```python
from build123d import *

# Parameters (mm, degrees)
F3_DEPTH = 30
F4_DEPTH = 30
F5_DEPTH = 30


with BuildPart() as f3:
    # F0 (on Top) → F3 (new body, symmetric)
    with BuildSketch(Plane.XY):
        Polygon((17.320508, 30), (-17.320508, 30), (-34.641016, 0), (-17.320508, -30), (17.320508, -30), (34.641016, 0), align=None)
    extrude(amount=F3_DEPTH, both=True)

    # F1 (on Right) → F4 (intersect, symmetric)
    with BuildSketch(Plane.YZ):
        Polygon((30, -17.320508), (30, 17.320508), (0, 34.641016), (-30, 17.320508), (-30, -17.320508), (0, -34.641016), align=None)
    extrude(amount=F4_DEPTH, both=True, mode=Mode.INTERSECT)

    # F2 (on Front) → F5 (intersect, symmetric)
    with BuildSketch(Plane.XZ):
        Polygon((17.320508, 30), (-17.320508, 30), (-34.641016, 0), (-17.320508, -30), (17.320508, -30), (34.641016, 0), align=None)
    extrude(amount=F5_DEPTH, both=True, mode=Mode.INTERSECT)


solid = f3.part
```
Model file for the job. Use its own axes, mm. Give positions to 0.01 mm unless a question says otherwise; leave off trailing zeros. Order: outer loops, then holes, each group sorted by start corner. A loop starts at its lowest first (then second) coordinate and runs counter-clockwise, first axis right, second up.
1) Saw through at A-A, the plane z = 3. Write the cut outline in (x, y).
2) Pin check, flat tips, straight feed: pin 1 (5 mm diameter, centred on x = 19.5, y = -19, fed in from +Z); pin 2 (4 mm diameter, centred on y = -13.5, z = -3.5, fed in from -X); pin 3 (3 mm diameter, centred on x = 8, y = -11.5, fed in from +Z). Stop position of each tip, or through.
3) Wall check: probe 1 along Y at (x, z) = (-20, 3); probe 2 along Y at (x, z) = (18, -21.5); probe 3 along X at (y, z) = (-5, 20). Give the ranges that are in metal, low to high.
4) Saw through at D-D, the plane z = 26. Write the cut outline in (x, y).
5) Saw through at C-C, the plane x = -23. Write the cut outline in (y, z), then the cut area to 3 significant figures.
Computed:
1. outline: (-30, -8.04) - (-17.32, -30) - (17.32, -30) - (30, -8.04) - (30, 8.04) - (17.32, 30) - (-17.32, 30) - (-30, 8.04) - close
2. pin 1: stops at z = 25.11
2. pin 2: stops at x = -28
2. pin 3: stops at z = 28.87
3. probe 1: y = -25.36 to 25.36
3. probe 2: y = -22.76 to 22.76
3. probe 3: x = -23.09 to 23.09
4. outline: (-19.63, -14.97) - (19.63, -14.97) - (19.63, 14.97) - (-19.63, 14.97) - close
5. outline: (-20.16, -20.16) - (20.16, -20.16) - (20.16, 20.16) - (-20.16, 20.16) - close
5. area: 1,630 mm2
